Design review of the part shown in the three views and the two pictorial views. Dimensions are in mm from the part's minimum x, y and z. A direction names the side the tool comes from. Coordinates: 2 decimals unless noted, no trailing zeros. Write each loop counter-clockwise with the first axis right and the second up, starting at its lowest first coordinate (ties: lowest second). Pieces come first, ordered by that corner, then holes. Notation, with made-up numbers: M 28,7.25 L 76,7.25 A32 ccw 76,40.25 Z; hole C 56,36 d10. An arc over 180 degrees is marked long. One line per question, with ' | ' between items.
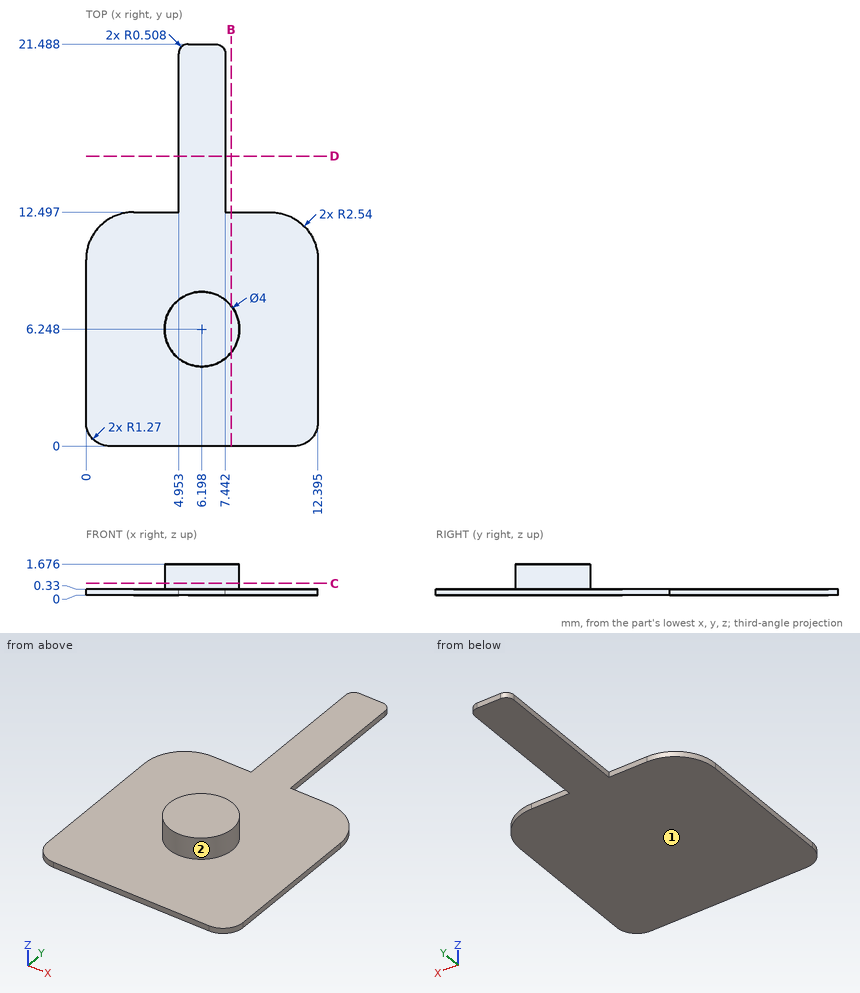
1. Take a section at B-B on x = 7.75. State the section outline as (y, z) points.
Computed values:
outline: M 0,0 L 12.5,0 L 12.5,0.33 L 7.51,0.33 L 7.51,1.68 L 4.99,1.68 L 4.99,0.33 L 0,0.33 Z
2. Take a section at C-C on z = 0.65. State the section outline as (x, y) points.
Computed values:
outline: C 6.2,6.25 d4
3. Machinability: for the marked faces 1 and 2, which of the approach directions +Z, -Z, +X, -X, +Y, -Y give a long, thin tool a straight path to every point of the face, cutting with its end or side? Answer none if there is none.
Computed values:
face 1: -Z, +X, -X, +Y, -Y | face 2: +Z
4. For line 1 along Z through (x, y) = (3.5, 8); line 2 along Y through (x, z) = (4.25, 0.2); line 3 along X through (y, z) = (18, 0.3), list the stretches that pass through material, from the lowest coordinate up.
Computed values:
line 1: z = 0 to 0.33 | line 2: y = 0 to 12.5 | line 3: x = 4.95 to 7.44
5. Take a section at D-D on y = 15.5. State the section outline as (x, z) points.
Computed values:
outline: M 4.95,0 L 7.44,0 L 7.44,0.33 L 4.95,0.33 Z
6. Clearance check with flat-ended pins moving along their axes: P1, Ø1, axis at y = 6.5, z = 1, coming from the +X side; P2, Ø1.5, axis at x = 9, y = 6, coming from the +Z side; P3, Ø1, axis at y = 14, z = 0.5, coming from the +X side. State where each tip first meets the part, or that it passes through.
Computed values:
P1: stops at x = 8.2 | P2: stops at z = 0.33 | P3: stops at x = 7.44
